from build123d import *

# Parameters (mm, degrees)
BOSS_EXTRUDE1_DEPTH = 15
CUT_EXTRUDE1_DEPTH  = 25


with BuildPart() as part:
    # Sketch1 → Boss-Extrude1 (new body)
    with BuildSketch(Plane(origin=(0, 0, 0), x_dir=(1, 0, 0), z_dir=(0, 1, 0))):
        with BuildLine():
            ThreePointArc((55.608003021, 10), (56.276558933, 5.019852055), (56.5, 0))
            ThreePointArc((56.5, 0), (56.276558933, -5.019852055), (55.608003021, -10))
            Line((55.608003021, -10), (57, -8.608003021))
            Line((57, -8.608003021), (57, 8.608003021))
            Line((57, 8.608003021), (55.608003021, 10))
        make_face()
    extrude(amount=BOSS_EXTRUDE1_DEPTH)

    # Sketch2 → Cut-Extrude1 (cut)
    with BuildSketch(Plane(origin=(67, 0, 0), x_dir=(0, 0, -1), z_dir=(1, 0, 0))):
        with BuildLine():
            ThreePointArc((0, 11.5), (-4, 7.5), (0, 3.5))
            Line((0, 3.5), (0, 11.5))
        make_face()
        with BuildLine():
            Line((0, 11.5), (0, 3.5))
            ThreePointArc((0, 3.5), (2.828427125, 4.671572875), (4, 7.5))
            ThreePointArc((4, 7.5), (2.828427125, 10.328427125), (0, 11.5))
        make_face()
    extrude(amount=-CUT_EXTRUDE1_DEPTH, mode=Mode.SUBTRACT)


solid = part.part
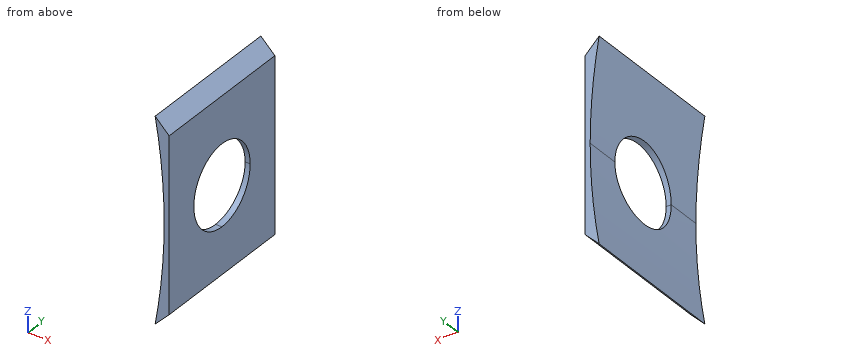
The listing builds one solid part. Answer for the finished solid, in the listing's coordinates (mm). Coordinates: 2 decimals unless noted, no trailing zeros. Loops run counter-clockwise (first coordinate to the right, second up) from the corner with the lowest first, then second, coordinate; pieces in that order, holes last.
1) Find section A-A on z = 3. Write down the section's boundary in (x, y), then the cut area to 3 significant figures.
2) Find section C-C on y = 12.25. Write down the section's boundary in (x, z), then the cut area to 3 significant figures.
3) A flat-ended cylindrical pin translates along its axis: pin 1 Ø8 at (y, z) = (4.5, -4) entering from -X. Find the tip coordinate at first contact, or state that the pin passes through.
4) Find section B-B on y = 4.25. Write down the section's boundary in (x, z).
5) Find the intervals of material crossed by L1, parallel to Y at x = 56.8, z = -1.75; L2, parallel to Z at x = 56.45, y = 9.25; L3, parallel to Z at x = 56.55, y = 4, in increasing order.
6) Find section D-D on z = -5.25. Write down the section's boundary in (x, y).
Values:
1. outline: (56.42, 0) - (57, 0) - (57, 4.85) - (56.42, 4.85) - close; (56.42, 10.15) - (57, 10.15) - (57, 15) - (56.42, 15) - close
1. area: 5.63 mm2
2. outline: (55.61, -10) - (57, -8.61) - (57, 8.61) - (55.61, 10) arc R56.5 cw to start
2. area: 14.0 mm2
3. pin 1: stops at x = 55.93
4. outline: (55.61, -10) - (57, -8.61) - (57, -2.33) - (56.45, -2.33) arc R56.5 cw to start; (55.61, 10) arc R56.5 cw to (56.45, 2.33) - (57, 2.33) - (57, 8.61) - close
5. L1: y = 0 to 3.9, 11.1 to 15
5. L2: z = -9.16 to -3.6, 3.6 to 9.16
5. L3: z = -9.06 to -1.94, 1.94 to 9.06
6. outline: (56.26, 0) - (57, 0) - (57, 15) - (56.26, 15) - close
